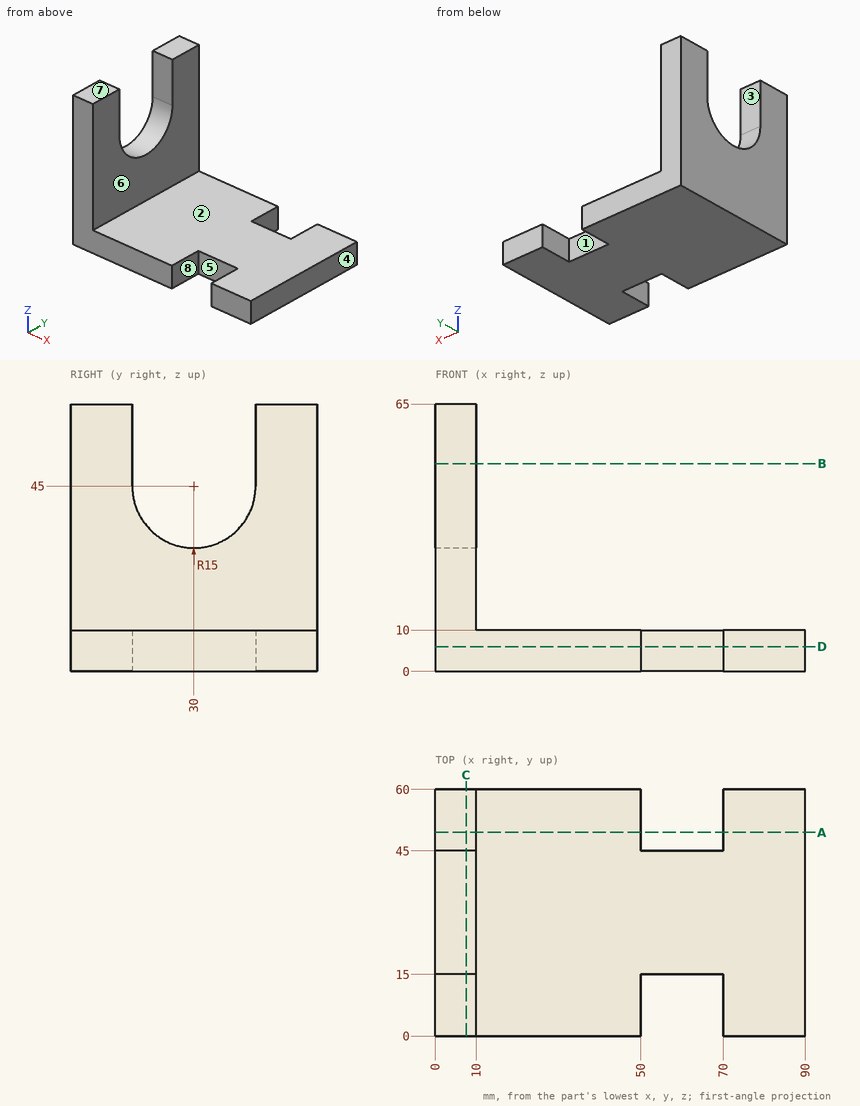
Study the drawing (mm; zero at the part's minimum x, y, z) and answer. A direction names the side the tool comes from. Coordinates: 2 decimals unless noted, no trailing zeros. Write each loop counter-clockwise with the first axis right and the second up, starting at its lowest first coordinate (ties: lowest second). Pieces come first, ordered by that corner, then holes. Notation, with made-up numbers: M 4,-7 L 40,-7 A25 ccw 40,20 Z; hole C 42.25,9 d8. An arc over 180 degrees is marked long. Use one line per item in the form item = value.
Item 1: Find section B-B, the plane z = 50.5. Give the vertices of the cut face in (x, y).
Model answer:
outline = M 0,0 L 10,0 L 10,15 L 0,15 Z; M 0,45 L 10,45 L 10,60 L 0,60 Z
Item 2: Given P1, Ø8, axis at y = 32, z = 23, coming from the +X side; P2, Ø12, axis at x = 40, y = 52.5, coming from the +Z side; P3, Ø8, axis at x = 57, z = 6.5, coming from the -Y side, each flat-ended and moving along its own axis, determine where each tip first touches the part or whether it passes through.
Model answer:
P1 = 10
P2 = 10
P3 = 15
Item 3: Find section C-C, the plane x = 7.5. Give the vertices of the cut face in (y, z).
Model answer:
outline = M 0,0 L 60,0 L 60,65 L 45,65 L 45,45 A15 cw 15,45 L 15,65 L 0,65 Z
Item 4: Find the intervals of material crossed by probe 1 along Z at (x, y) = (83.5, 55.5), in increasing order.
Model answer:
probe_1 = 0 to 10
Item 5: For the marked faces 1, 2, 3, 4 and 5, determine the directions among +Z, -Z, +X, -X, +Y, -Y from which every point of the face is accessible in a straight line to the end or side of a thin tool.
Model answer:
face_1 = +Z, -Z, +Y
face_2 = +Z, +X, +Y, -Y
face_3 = +Z, +X, -X
face_4 = +Z, -Z, +X, +Y, -Y
face_5 = +Z, -Z, -Y
Item 6: The mould has two halves that part along X. Classify the marked faces 6, 7 and 8: released by +X, released by -X, zero draft, split by the parting line, or undercut.
Model answer:
face_6 = released by +X
face_7 = zero draft
face_8 = undercut
Item 7: Find section D-D, the plane z = 6. Give the vertices of the cut face in (x, y).
Model answer:
outline = M 0,0 L 50,0 L 50,15 L 70,15 L 70,0 L 90,0 L 90,60 L 70,60 L 70,45 L 50,45 L 50,60 L 0,60 Z
Item 8: Find section A-A, the plane y = 49.5. Give the vertices of the cut face in (x, z).
Model answer:
outline = M 0,0 L 50,0 L 50,10 L 10,10 L 10,65 L 0,65 Z; M 70,0 L 90,0 L 90,10 L 70,10 Z
